```python
from build123d import *

# Parameters (mm, degrees)
SKETCH1_W           = 499
SKETCH1_H           = 18
SKETCH1_W_2         = 18
SKETCH1_H_2         = 64
BOSS_EXTRUDE1_DEPTH = 515
SKETCH4_W           = 699
SKETCH4_H           = 533
BOSS_EXTRUDE2_DEPTH = 18
SKETCH5_W           = 699
SKETCH5_H           = 533
BOSS_EXTRUDE3_DEPTH = 18
SKETCH7_W           = 18
SKETCH7_H           = 351
BOSS_EXTRUDE4_DEPTH = 50
SKETCH8_W           = 18
SKETCH8_H           = 351
BOSS_EXTRUDE5_DEPTH = 50
SKETCH9_R           = 152.5
CUT_EXTRUDE1_DEPTH  = 50


with BuildPart() as part:
    # Sketch1 → Boss-Extrude1 (new body)
    with BuildSketch(Plane(origin=(0, 0, 0), x_dir=(1, 0, 0), z_dir=(0, 1, 0))):
        Polygon((249.5, -272.327471245), (331.5, -272.327471245), (331.5, 224.672528755), (-331.5, 224.672528755), (-331.5, -272.327471245), (-249.5, -272.327471245), (-249.5, -290.327471245), (-349.5, -290.327471245), (-349.5, 242.672528755), (349.5, 242.672528755), (349.5, -290.327471245), (249.5, -290.327471245), align=None)
        Polygon((249.5, -208.327471245), (267.5, -208.327471245), (267.5, 160.672528755), (72.5, 160.672528755), (72.5, 142.672528755), (249.5, 142.672528755), align=None)
        with Locations((0, 69.672528755)):
            Rectangle(SKETCH1_W, SKETCH1_H)
        with Locations((0, 192.672528755)):
            Rectangle(SKETCH1_W_2, SKETCH1_H_2)
        Polygon((-249.5, -208.327471245), (-267.5, -208.327471245), (-267.5, 160.672528755), (-72.5, 160.672528755), (-72.5, 142.672528755), (-249.5, 142.672528755), align=None)
    extrude(amount=BOSS_EXTRUDE1_DEPTH)

    # Sketch4 → Boss-Extrude2 (add)
    with BuildSketch(Plane(origin=(0, 0, 0), x_dir=(1, 0, 0), z_dir=(0, 1, 0))):
        with Locations((0, -23.827471245)):
            Rectangle(SKETCH4_W, SKETCH4_H)
    extrude(amount=BOSS_EXTRUDE2_DEPTH)

    # Sketch5 → Boss-Extrude3 (add)
    with BuildSketch(Plane(origin=(0, 515, 0), x_dir=(1, 0, 0), z_dir=(0, 1, 0))):
        with Locations((0, -23.827471245)):
            Rectangle(SKETCH5_W, SKETCH5_H)
    extrude(amount=BOSS_EXTRUDE3_DEPTH)

    # Sketch7 → Boss-Extrude4 (add)
    with BuildSketch(Plane(origin=(0, 18, 0), x_dir=(1, 0, 0), z_dir=(0, 1, 0))):
        with Locations((63.5, -114.827471245)):
            Rectangle(SKETCH7_W, SKETCH7_H)
        with Locations((-63.5, -114.827471245)):
            Rectangle(SKETCH7_W, SKETCH7_H)
    extrude(amount=BOSS_EXTRUDE4_DEPTH)

    # Sketch8 → Boss-Extrude5 (add)
    with BuildSketch(Plane.XZ.offset(-515)):
        with Locations((-63.5, 114.827471245)):
            Rectangle(SKETCH8_W, SKETCH8_H)
        with Locations((63.5, 114.827471245)):
            Rectangle(SKETCH8_W, SKETCH8_H)
    extrude(amount=BOSS_EXTRUDE5_DEPTH)

    # Sketch9 → Cut-Extrude1 (cut)
    with BuildSketch(Plane.XY.offset(-60.672528755)):
        with Locations((0, 266.5)):
            Circle(SKETCH9_R)
    extrude(amount=-CUT_EXTRUDE1_DEPTH, mode=Mode.SUBTRACT)


solid = part.part
```
Geometry check sheet. Reference: the model listing, model coordinates, mm. A direction names the side the tool comes from. Give positions to 0.01 mm unless a question says otherwise; leave off trailing zeros. Order: outer loops, then holes, each group sorted by start corner. A loop starts at its lowest first (then second) coordinate and runs counter-clockwise, first axis right, second up. Notation, with made-up numbers: (32, 21) - (38, 21) arc R21 ccw to (38, 57) - close; hole circle Ø4 at (85, -37.5). An arc over 180 degrees is marked (long way). Answer in a Markdown table with one row per item. Add a question column.
Q1. Cross-section at B-B, the plane x = -239. Enter the section's corners in (y, z), then the cut area to 3 significant figures.
Q2. Material ranges on probe 1 along Z at (x, y) = (-261.5, 464.5); probe 2 along Z at (x, y) = (-239, 379); probe 3 along X at (y, z) = (266, -70), recorded low to high. Write a range as from..to.
Q3. Cross-section at A-A, the plane z = -88.5. Enter the section's corners in (x, y).
Q4. Cross-section at D-D, the plane x = -87. Enter the section's corners in (y, z), then the cut area to 3 significant figures.
Q5. Gauge pin test, flat end, axial feed: pin 1 (10 mm diameter, centred on x = -50, y = 201.5, fed in from +Z). Record the tip position at first contact, or that the pin passes through.
Q6. Tool access check on faces 1 (the flat face through (-5, 263, -242.673)), 2 (the flat face through (-64, 465, 117)), 3 (the flat face through (290, 263, 272.327)). Record the directions out of +Z, -Z, +X, -X, +Y, -Y that give a thin tool (end or side, any length) a straight path to the whole face; none if there is none.
Q7. Mould release check, pull along Y, two halves, no side actions. Record for faces 4 (the flat face through (-349.5, 263, 28)), 5 (the flat face through (-54.5, 490, 112)), 6 (the flat face through (-72.5, 263, -152)): pulls with the +Y half, pulls with the -Y half, needs draft (parallel to the pull), parting line crosses it, or undercut.
Q8. Cross-section at C-C, the plane y = 266.5. Count the separate pieces of the cut face and the enclosed holes in it, then the cut area to 3 significant figures.
Check values:
| question | item | result |
|---|---|---|
| 1 | outline | (0, -242.67) - (533, -242.67) - (533, 290.33) - (515, 290.33) - (515, -60.67) - (18, -60.67) - (18, 290.33) - (0, 290.33) - close; hole (18, -224.67) - (515, -224.67) - (515, -160.67) - (18, -160.67) - close; hole (18, -142.67) - (515, -142.67) - (515, -78.67) - (18, -78.67) - close |
| 1 | area | 46,000 mm^2 |
| 2 | probe 1 | z = -242.67..-224.67, -160.67..208.33, 272.33..290.33 |
| 2 | probe 2 | z = -242.67..-224.67, -160.67..-142.67, -78.67..-60.67 |
| 2 | probe 3 | x = -349.5..-331.5, -267.5..-152.5, 152.5..267.5, 331.5..349.5 |
| 3 | outline | (-349.5, 0) - (349.5, 0) - (349.5, 533) - (-349.5, 533) - close; hole (-331.5, 18) - (-267.5, 18) - (-267.5, 515) - (-331.5, 515) - close; hole (-249.5, 18) - (249.5, 18) - (249.5, 515) - (-249.5, 515) - close; hole (267.5, 18) - (331.5, 18) - (331.5, 515) - (267.5, 515) - close |
| 4 | outline | (0, -242.67) - (533, -242.67) - (533, 290.33) - (515, 290.33) - (515, -60.67) - (391.75, -60.67) - (391.75, -78.67) - (515, -78.67) - (515, -142.67) - (18, -142.67) - (18, -78.67) - (141.25, -78.67) - (141.25, -60.67) - (18, -60.67) - (18, 290.33) - (0, 290.33) - close; hole (18, -224.67) - (515, -224.67) - (515, -160.67) - (18, -160.67) - close |
| 4 | area | 41,500 mm^2 |
| 5 | pin 1 | stops at z = -224.67 |
| 6 | face 1 | -Z, +X, -X, +Y, -Y |
| 6 | face 2 | +Z |
| 6 | face 3 | none |
| 7 | face 4 | needs draft |
| 7 | face 5 | undercut |
| 7 | face 6 | undercut |
| 8 | separate pieces | 3 |
| 8 | enclosed holes | 0 |
| 8 | area | 58,400 mm^2 |
